Design review of the part built by this model. Coordinates are the model's own, in mm. A direction names the side the tool comes from. Coordinates: 2 decimals unless noted, no trailing zeros. Loops run counter-clockwise (first coordinate to the right, second up) from the corner with the lowest first, then second, coordinate; pieces in that order, holes last. Notation, with made-up numbers: (18.5, -25) -> (61.5, -25) arc R28 ccw to (61.5, -4) -> close; hole circle Ø6 at (5, 45). An arc over 180 degrees is marked (long way). Use one line per item in the form item = value. Start each with the question number.
1. Wall thickness on line 1 (X direction, y = 30, z = 3.75); line 2 (X direction, y = 9, z = 8); line 3 (Y direction, x = -16, z = 15.25): over which ranges is each line inside the solid? List them lowest first. Write a range as from..to.
2. For pin 1 (3.5 mm diameter, centred on y = 29.5, z = 14, fed in from -X); pin 2 (6 mm diameter, centred on y = 19, z = 2, fed in from -X); pin 3 (1.5 mm diameter, centred on x = 4.5, z = 16, fed in from -Y), all flat-tipped, find the tip position at first contact; note any pin that passes through.
3. Consider section A-A (z = 3.5). State the section outline as (x, y) points.
4. Machinability: for faces 1 (the face through (-22.6, 0, 9)), 2 (the face through (-17, 9.6, 9)), which of the approach directions +Z, -Z, +X, -X, +Y, -Y give a long, thin tool a straight path to every point of the face, cutting with its end or side? Answer none if there is none.
5. Consider section C-C (x = -14). State the section outline as (y, z) points.
6. Consider section B-B (y = 31.5). State the section outline as (x, z) points, then the cut area to 3 significant figures.
from build123d import *

# Parameters (mm, degrees)
F0_W     = 19.2
F0_H     = 19.2
F0_W_2   = 26
F0_H_2   = 26
F1_DEPTH = 19.2
F2_R     = 14
F3_R     = 33.2


with BuildPart() as f1:
    # F0 (on Top) → F1 (new body)
    with BuildSketch(Plane.XY):
        with Locations((13, 0)):
            Rectangle(F0_W, F0_H)
        with Locations((-9.6, 0)):
            Rectangle(F0_W_2, F0_H)
        with Locations((13, 22.6)):
            Rectangle(F0_W, F0_H_2)
    extrude(amount=F1_DEPTH)

    # F2
    f2_edges = [f1.edges().sort_by_distance(p)[0] for p in [
        (3.4, 9.6, 9.6),
    ]]
    fillet(f2_edges, radius=F2_R)

    # F3
    f3_edges = [f1.edges().sort_by_distance(p)[0] for p in [
        (22.6, -9.6, 9.6),
    ]]
    fillet(f3_edges, radius=F3_R)


solid = f1.part
Geometry check:
q1.line_1 = 3.4..22.6
q1.line_2 = -22.6..19.22
q1.line_3 = -9.6..9.6
q2.pin_1 = 3.4
q2.pin_2 = 1.16
q2.pin_3 = -6.34
q3.outline = (-22.6, -9.6) -> (-10.6, -9.6) arc R33.2 ccw to (22.6, 23.6) -> (22.6, 35.6) -> (3.4, 35.6) -> (3.4, 23.6) arc R14 cw to (-10.6, 9.6) -> (-22.6, 9.6) -> close
q4.face_1 = +Z, -Z, -X, +Y, -Y
q4.face_2 = +Z, -Z, -X, +Y
q5.outline = (-9.6, 0) -> (9.6, 0) -> (9.6, 19.2) -> (-9.6, 19.2) -> close
q6.outline = (3.4, 0) -> (22.6, 0) -> (22.6, 19.2) -> (3.4, 19.2) -> close
q6.area = 369 mm²
